For this review, use the dimensioned drawing (mm, ordinates from the lowest corner) and the shaded views. Give positions to 0.01 mm unless a question says otherwise; leave off trailing zeros. Order: outer loops, then holes, each group sorted by start corner. A loop starts at its lowest first (then second) coordinate and runs counter-clockwise, first axis right, second up. Notation, with made-up numbers: (8.25, 81) -> (66.25, 81) arc R25 ccw to (66.25, 100) -> close; hole circle Ø2 at (54.25, 24). An arc over 180 degrees is marked (long way). One line per item, written item: value. Start each with the question number.
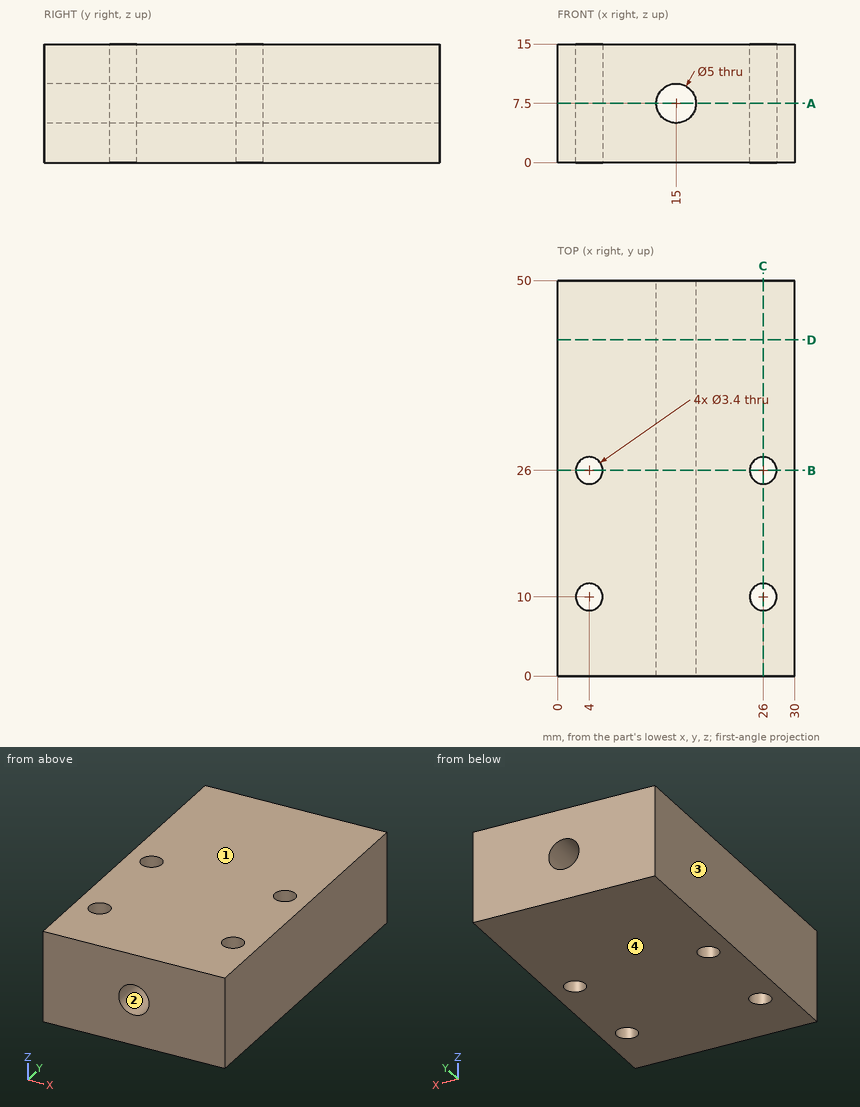
Q1. Take a section at D-D (y = 42.5). State the section outline as (x, z) points, and give its area (3 significant figures).
Q2. Mouldability with a two-part tool opening along Z and no side actions: class the marked faces 1, 2, 3 and 4 as pulls with the +Z half, pulls with the -Z half, needs draft (parallel to the pull), parting line crosses it, or undercut.
Q3. Take a section at A-A (z = 7.5). State the section outline as (x, y) points.
Q4. For line 1 along Y through (x, z) = (4, 10.75); line 2 along X through (y, z) = (11.5, 9.25); line 3 along Z through (x, y) = (15, 25.5), list the stretches that pass through material, from the lowest coordinate up.
Q5. Take a section at C-C (x = 26). State the section outline as (y, z) points, and give its area (3 significant figures).
Q6. Take a section at B-B (y = 26). State the section outline as (x, z) points.
Answers below:
1. outline: (0, 0) -> (30, 0) -> (30, 15) -> (0, 15) -> close; hole circle Ø5 at (15, 7.5)
1. area: 430 mm²
2. face 1: pulls with the +Z half
2. face 2: undercut
2. face 3: needs draft
2. face 4: pulls with the -Z half
3. outline: (0, 0) -> (12.5, 0) -> (12.5, 50) -> (0, 50) -> close; (17.5, 0) -> (30, 0) -> (30, 50) -> (17.5, 50) -> close; hole circle Ø3.4 at (4, 10); hole circle Ø3.4 at (4, 26); hole circle Ø3.4 at (26, 10); hole circle Ø3.4 at (26, 26)
4. line 1: y = 0 to 8.3, 11.7 to 24.3, 27.7 to 50
4. line 2: x = 0 to 3.2, 4.8 to 13.21, 16.79 to 25.2, 26.8 to 30
4. line 3: z = 0 to 5, 10 to 15
5. outline: (0, 0) -> (8.3, 0) -> (8.3, 15) -> (0, 15) -> close; (11.7, 0) -> (24.3, 0) -> (24.3, 15) -> (11.7, 15) -> close; (27.7, 0) -> (50, 0) -> (50, 15) -> (27.7, 15) -> close
5. area: 648 mm²
6. outline: (0, 0) -> (2.3, 0) -> (2.3, 15) -> (0, 15) -> close; (5.7, 0) -> (24.3, 0) -> (24.3, 15) -> (5.7, 15) -> close; (27.7, 0) -> (30, 0) -> (30, 15) -> (27.7, 15) -> close; hole circle Ø5 at (15, 7.5)
